Autodesk Inventor part; units mm, degrees
ref_plane "YZ Plane" through (0, 0, 0) normal (1, 0, 0) x (0, 1, 0)
ref_plane "XZ Plane" through (0, 0, 0) normal (0, 1, 0) x (-1, 0, 0)
ref_plane "XY Plane" through (0, 0, 0) normal (0, 0, 1) x (1, 0, 0)
sketch "Sketch1" plane through (0, 0, 0) normal (0, 1, 0) x (-1, 0, 0)
  line L0 (14, 0) -> (-14, 0)
  line L1 (0, -32.2) -> (0, 32.2)
  line L2 (10, 23) -> (-10, 23)
  line L3 (-10, 23) -> (-10, -23)
  line L4 (-10, -23) -> (10, -23)
  line L5 (10, -23) -> (10, 23)
  point P0 (0, 0)
  dimension "d0" = 46
  dimension "d1" = 20
extrude "Extrusion1" add sketch "Sketch1" along normal blind 4
sketch "Sketch2" plane through (0, 4, 0) normal (0, 1, 0) x (1, 0, 0)
  line L0 (-10, -23) -> (10, -23)
  line L1 (10, -23) -> (10, 23)
  line L2 (10, 23) -> (-10, 23)
  line L3 (-10, 23) -> (-10, -23)
  line L4 (-10, -23) -> (10, -23)
  line L5 (10, -23) -> (10, -19)
  line L6 (10, -19) -> (-10, -19)
  line L7 (-10, -19) -> (-10, -23)
  line L8 (-10, 19) -> (10, 19)
  line L9 (10, 19) -> (10, 23)
  line L10 (10, 23) -> (-10, 23)
  line L11 (-10, 23) -> (-10, 19)
  line L12 (-10, -23) -> (10, -23)
  line L13 (-10, 23) -> (-10, -23)
  line L14 (10, -23) -> (10, 23)
  line L15 (10, 23) -> (-10, 23)
  point P0 (0, 0)
  dimension "d4" = 4
  dimension "d5" = 4
extrude "Extrusion2" add sketch "Sketch2" along normal blind 30 contours L3 L6 L1 L0 | L3 L2 L1 L8
sketch "Sketch4" plane through (-10, 0, 23) normal (0, 0, 1) x (1, 0, 0)
  line L0 (0, 0) -> (20, 0)
  line L1 (20, 0) -> (20, 34)
  line L2 (0, 34) -> (20, 34)
  line L3 (0, 0) -> (0, 34)
  point P0 (10, 0)
  point P1 (10, 26)
  dimension "d8" = 10
  dimension "d9" = 8
hole "Hole1" at (0, 26, 23) direction (0, 0, -1) diameter 8 depth 42
sketch "Sketch10" plane through (10, 0, -23) normal (0, 0, -1) x (-1, 0, 0)
  line L0 (0, 34) -> (20, 34)
  line L1 (0, 0) -> (0, 34)
  line L2 (0, 0) -> (20, 0)
  line L3 (20, 0) -> (20, 34)
  circle A0 centre (10, 26) radius 4
  circle A1 centre (10, 26) radius 3.75
  circle A2 centre (10, 12) radius 2.5
  line L4 (-6.7241, 9.5) -> (37.2046, 9.5) construction
  line L5 (6.25, 26) -> (7.5505, 11.5)
  line L6 (13.75, 26) -> (12.4495, 11.5)
  point P0 (10, 0)
  dimension "d47" = 16.5
  dimension "d48" = 7.5
  dimension "d49" = 5
  dimension "d50" = 10
  dimension "d51" = 2
  dimension "d52" = 2
  dimension "d53" = 8
  dimension "d54" = 8
extrude "Extrusion4" cut sketch "Sketch10" against normal blind 2 contours L5 A1 L6 A0 | A0 L6 A2 L5 | L5 A1 L6 | A2 L6 L5 picked at (10.4522, 22.2104)
sketch "Sketch11" plane through (10, 0, -21) normal (0, 0, -1) x (-1, 0, 0)
  line L0 (7.5505, 11.5) -> (6.25, 26)
  arc A0 (7.5505, 11.5) -> (12.4495, 11.5) centre (10, 12) ccw
  line L1 (13.75, 26) -> (12.4495, 11.5)
  arc A1 (13.75, 26) -> (6.25, 26) centre (10, 26) ccw
  point P0 (10, 0)
hole "Hole4" at (0, 26, -21) direction (0, 0, 1) diameter 7.5 depth 40
sketch "Sketch12" plane through (10, 0, -21) normal (0, 0, -1) x (-1, 0, 0)
  arc A0 (6.3099, 25.3327) -> (13.6901, 25.3327) centre (10, 26) ccw
  line L0 (7.5505, 11.5) -> (6.3099, 25.3327)
  arc A1 (7.5505, 11.5) -> (12.4495, 11.5) centre (10, 12) ccw
  line L1 (13.6901, 25.3327) -> (12.4495, 11.5)
  line L2 (0, 0) -> (0, 34)
  point P0 (10, 0)
  point P1 (10, 19.5)
  point P2 (0, 28)
  dimension "d64" = 6.5
  dimension "d65" = 10
hole "Hole5" at (0, 19.5, -21) direction (0, 0, 1) diameter 2.5 depth 40
sketch "Sketch13" plane through (0, 0, 0) normal (0, -1, 0) x (1, 0, 0)
  line L0 (-10, 23) -> (10, 23)
  line L1 (-10, -23) -> (-10, 23)
  line L2 (10, -23) -> (-10, -23)
  line L3 (10, 23) -> (10, -23)
  line L4 (10, 23) -> (10, -23)
  line L5 (-10, -19) -> (-10, 19)
  line L6 (10, 23) -> (-10, 23)
  line L7 (-10, 23) -> (-10, 19)
  line L8 (-10, 19) -> (10, 19)
  line L9 (10, 19) -> (10, 23)
  line L10 (10, -23) -> (-10, -23)
  line L11 (-10, -23) -> (-10, -19)
  line L12 (-10, -19) -> (10, -19)
  line L13 (10, -19) -> (10, -23)
  point P0 (0, 0)
extrude "Extrusion5" add sketch "Sketch13" along normal blind 30 contours L0 L3 L8 L1 | L12 L3 L2 L1
sketch "Sketch14" plane through (10, 34, -23) normal (0, 0, -1) x (-1, 0, 0)
  arc A0 (7.5505, -22.5) -> (12.4495, -22.5) centre (10, -22) ccw
  line L0 (7.5505, -22.5) -> (6.25, -8)
  arc A1 (13.75, -8) -> (6.25, -8) centre (10, -8) ccw
  line L1 (13.75, -8) -> (12.4495, -22.5)
  line L2 (20, -64) -> (20, 0)
  line L3 (0, 0) -> (20, 0)
  line L4 (0, -64) -> (0, 0)
  line L5 (20, -64) -> (0, -64)
  line L6 (0, -34) -> (0, -64)
  line L7 (0, -40) -> (20, -40) construction
  circle A2 centre (10, -56) radius 3.75
  circle A3 centre (10, -42.5) radius 2.5
  line L8 (6.25, -56) -> (7.5505, -42)
  line L9 (13.75, -56) -> (12.4495, -42)
  point P0 (10, -34)
  dimension "d77" = 8
  dimension "d78" = 10
  dimension "d79" = 7.5
  dimension "d80" = 16
  dimension "d81" = 5
  dimension "d82" = 10
  dimension "d85" = 2
  dimension "d86" = 8
  dimension "d87" = 2
  dimension "d88" = 8
extrude "Extrusion6" cut sketch "Sketch14" against normal blind 2 contours L8 A2 L9 | L8 A3 L9 A2 | L8 A3 L9
sketch "Sketch15" plane through (10, 34, -21) normal (0, 0, -1) x (-1, 0, 0)
  arc A0 (6.25, -56) -> (13.75, -56) centre (10, -56) ccw
  line L0 (12.4495, -42) -> (13.75, -56)
  arc A1 (12.4495, -42) -> (7.5505, -42) centre (10, -42.5) ccw
  line L1 (6.25, -56) -> (7.5505, -42)
  point P0 (10, -34)
hole "Hole6" at (0, -22, -21) direction (0, 0, 1) diameter 7.5 depth 40
sketch "Sketch16" plane through (10, 34, -21) normal (0, 0, -1) x (-1, 0, 0)
  arc A0 (13.6858, -55.3093) -> (6.3142, -55.3093) centre (10, -56) ccw
  line L0 (12.4495, -42) -> (13.6858, -55.3093)
  arc A1 (12.4495, -42) -> (7.5505, -42) centre (10, -42.5) ccw
  line L1 (6.3142, -55.3093) -> (7.5505, -42)
  line L2 (12.4495, -42) -> (13.75, -56)
  arc A2 (6.25, -56) -> (13.75, -56) centre (10, -56) ccw
  line L3 (6.25, -56) -> (7.5505, -42)
  arc A3 (12.4495, -42) -> (7.5505, -42) centre (10, -42.5) ccw
  arc A4 (7.5505, -22.5) -> (12.4495, -22.5) centre (10, -22) ccw
  line L4 (7.5505, -22.5) -> (6.25, -8)
  arc A5 (13.75, -8) -> (6.25, -8) centre (10, -8) ccw
  line L5 (13.75, -8) -> (12.4495, -22.5)
  line L6 (20, -64) -> (20, 0)
  line L7 (0, 0) -> (20, 0)
  line L8 (0, -64) -> (0, 0)
  line L9 (20, -64) -> (0, -64)
  point P0 (10, -34)
  point P1 (10, -49.5)
  dimension "d98" = 10
  dimension "d99" = 6.5
hole "Hole7" at (0, -15.5, -21) direction (0, 0, 1) diameter 2.5 end up to surface
sketch "Sketch17" plane through (-10, 34, 23) normal (0, 0, 1) x (1, 0, 0)
  line L0 (20, -64) -> (0, -64)
  line L1 (20, -64) -> (20, 0)
  point P0 (10, -34)
  point P1 (10, -56)
  dimension "d107" = 8
  dimension "d108" = 10
hole "Hole8" at (0, -22, 23) direction (0, 0, -1) diameter 8 depth 4
fillet "Fillet4" radius 6 8 edges at (10, -30, -21) (-10, -30, -21) (10, -30, 21) (-10, -30, 21) (10, 34, 21) (10, 34, -21) (-10, 34, -21) (-10, 34, 21)
sketch "Sketch19" plane through (0, 0, 0) normal (0, -1, 0) x (1, 0, 0)
  line L0 (10, 19) -> (-10, 19)
  line L1 (-10, -19) -> (-10, 19)
  line L2 (-10, -19) -> (10, -19)
  line L3 (10, 19) -> (10, -19)
  line L4 (-10, -19) -> (-10, 19)
  line L5 (10, 19) -> (-10, 19)
  line L6 (-10, -19) -> (0, -19)
  line L7 (0, -19) -> (0, 19)
  line L8 (0, 19) -> (-10, 19)
  line L9 (-10, 19) -> (-10, -19)
  point P0 (0, 0)
extrude "Extrusion8" cut sketch "Sketch19" against normal up to next contours L7 L2 L1 L0
chamfer "Chamfer1" distance 10 angle 45 2 edges at (0, 2, -19) (0, 2, 19)
fillet "Fillet6" radius 8 2 edges at (0, 2, 9) (0, 2, -9)
properties part number "v5_femur"
Design review of the part built by this model. Coordinates are the model's own, in mm. A direction names the side the tool comes from. Coordinates: 2 decimals unless noted, no trailing zeros. Order: outer loops, then holes, each group sorted by start corner. A loop starts at its lowest first (then second) coordinate and runs counter-clockwise, first axis right, second up.
Item 1: Take a section at D-D, the plane x = 4.75. Write out the cut boundary in (y, z).
Item 2: Take a section at B-B, the plane x = -6. Write out the cut boundary in (y, z).
Item 3: Take a section at A-A, the plane y = 6.5. Write out the cut boundary in (x, z), then the cut area to 3 significant figures.
Item 4: Take a section at C-C, the plane y = 19.5. Write out the cut boundary in (x, z), then the cut area to 3 significant figures.
Item 5: For pin 1 Ø12 at (x, z) = (1.5, -5) entering from -Y; pin 2 Ø10 at (x, z) = (3, 3) entering from +Y; pin 3 Ø4.5 at (y, z) = (2, 1) entering from -X; pin 4 Ø5 at (x, z) = (-6.5, -11) entering from -Y, all flat-tipped, find the tip position at first contact; note any pin that passes through.
Item 6: For faces 4 (the flat face through (2, 0, 0)), 5 (the flat face through (0, 16, -21)), 6 (the cylindrical face through (2.4, 29.2, 21)), list the 3-axis set-ups (+Z, -Z, +X, -X, +Y, -Y) from which the entire face can be reached by the end or side of a thin tool; tool diameter is ignored.
Item 7: The part is to be moulded in two halves that separate along Z. For faces 1 (the flat face through (0, 2, 23)), 2 (the cylindrical face through (-0.592, 2.028, -8.707)), 3 (the flat face through (-10, 2, -21)), say which applies: pulls with the +Z half, pulls with the -Z half, needs draft (parallel to the pull), parting line crosses it, or undercut.
Item 8: For line 1 (Y direction, x = 0, z = -20); line 2 (Y direction, x = 0, z = 21.4); line 3 (Z direction, x = -5, y = -5), list the stretches that pass through material, from the lowest coordinate up.
The answers:
1. outline: (-29.95, -23) - (33.95, -23) - (33.95, -19) - (4, -19) - (4, 19) - (33.95, 19) - (33.95, 23) - (-29.95, 23) - (-29.95, 19) - (0, 19) - (0, -19) - (-29.95, -19) - close
2. outline: (-29.66, -23) - (33.66, -23) - (33.66, -19) - (4, -19) - (4, -15) - (0, -15) - (0, -19) - (-29.66, -19) - close; (-29.66, 19) - (0, 19) - (0, 15) - (4, 15) - (4, 19) - (33.66, 19) - (33.66, 23) - (-29.66, 23) - close
3. outline: (-10, -23) - (10, -23) - (10, -19) - (-10, -19) - close; (-10, 19) - (10, 19) - (10, 23) - (-10, 23) - close
3. area: 160 mm2
4. outline: (-10, -23) - (-3.17, -23) - (-3.17, -21) - (-1.25, -21) - (-1.25, -19) - (-10, -19) - close; (-10, 19) - (10, 19) - (10, 23) - (-10, 23) - close; (1.25, -21) - (3.17, -21) - (3.17, -23) - (10, -23) - (10, -19) - (1.25, -19) - close
4. area: 142 mm2
5. pin 1: stops at y = 0
5. pin 2: stops at y = 4
5. pin 3: stops at x = 0
5. pin 4: passes through
6. face 4: +X, -X, -Y
6. face 5: -Z
6. face 6: +Z
7. face 1: pulls with the +Z half
7. face 2: undercut
7. face 3: needs draft
8. line 1: y = -30 to -25.75, -18.25 to -16.75, -14.25 to 18.25, 20.75 to 22.25, 29.75 to 34
8. line 2: y = -30 to -26, -18 to 22, 30 to 34
8. line 3: z = -23 to -19, 19 to 23
